```python
from build123d import *

# Parameters (mm, degrees)
F0_W     = 23.5877633095
F0_H     = 70.452131331
F0_R     = 11.8720680475
F1_DEPTH = 6


# Not quite as in the source:
# - a feature names something its author has since deleted; it is built from what else it names


with BuildPart() as f1:
    # F0 (on Front) → F1 (new body)
    with BuildSketch(Plane.XZ):
        with BuildLine():
            add(Edge.make_bspline(
                [(611.5972634537, -153.9022508941), (611.6433594367, -147.41064865), (611.6495089066, -143.6068529658), (611.6564787513, -143.3067750725)],
                knots=[235.725136676, 235.725136676, 235.725136676, 235.725136676, 267.1722290958, 267.1722290958, 267.1722290958, 267.1722290958], degree=3))
            Line((611.6564787513, -143.3067750725), (582.1564787513, -143.3067750725))
            Line((582.1564787513, -143.3067750725), (582.1564787513, -148.3067750725))
            Line((582.1564787513, -148.3067750725), (552.6564787513, -148.3067750725))
            Line((552.6564787513, -148.3067750725), (552.6564787513, -389.3067750725))
            Line((552.6564787513, -389.3067750725), (562.6564787513, -389.3067750725))
            Line((562.6564787513, -389.3067750725), (562.6564787513, -409.3067750725))
            Line((562.6564787513, -409.3067750725), (586.6564787513, -409.3067750725))
            add(Edge.make_bspline(
                [(586.6564787513, -409.3067750725), (608.6616471129, -402.2484026518), (611.2517312901, -202.5628331126), (611.5972634537, -153.9022508941)],
                knots=[0, 0, 0, 0, 235.725136676, 235.725136676, 235.725136676, 235.725136676], degree=3))
        make_face()
        with Locations((574.0745894078, -343.064654055)):
            Rectangle(F0_W, F0_H, mode=Mode.SUBTRACT)
        with Locations((580.0634622574, -230.3008177464)):
            Circle(F0_R, mode=Mode.SUBTRACT)
        with BuildLine():
            add(Edge.make_bspline(
                [(586.6564787513, 122.6932249275), (608.6616471129, 115.6348525069), (611.2517312901, -84.0507170322), (611.5972634537, -132.7112992508)],
                knots=[0, 0, 0, 0, 235.725136676, 235.725136676, 235.725136676, 235.725136676], degree=3))
            Line((586.6564787513, 122.6932249275), (562.6564787513, 122.6932249275))
            Line((562.6564787513, 122.6932249275), (562.6564787513, 102.6932249275))
            Line((562.6564787513, 102.6932249275), (552.6564787513, 102.6932249275))
            Line((552.6564787513, 102.6932249275), (552.6564787513, -138.3067750725))
            Line((552.6564787513, -138.3067750725), (582.1564787513, -138.3067750725))
            Line((582.1564787513, -138.3067750725), (582.1564787513, -143.3067750725))
            Line((582.1564787513, -143.3067750725), (611.6564787513, -143.3067750725))
            add(Edge.make_bspline(
                [(611.5972634537, -132.7112992508), (611.6433594367, -139.2029014949), (611.6495089066, -143.0066971792), (611.6564787513, -143.3067750725)],
                knots=[235.725136676, 235.725136676, 235.725136676, 235.725136676, 267.1722290958, 267.1722290958, 267.1722290958, 267.1722290958], degree=3))
        make_face()
        with Locations((580.0634622574, -56.3127323985)):
            Circle(F0_R, mode=Mode.SUBTRACT)
        with Locations((574.0745894078, 56.4511039101)):
            Rectangle(F0_W, F0_H, mode=Mode.SUBTRACT)
    extrude(amount=F1_DEPTH)


solid = f1.part
```
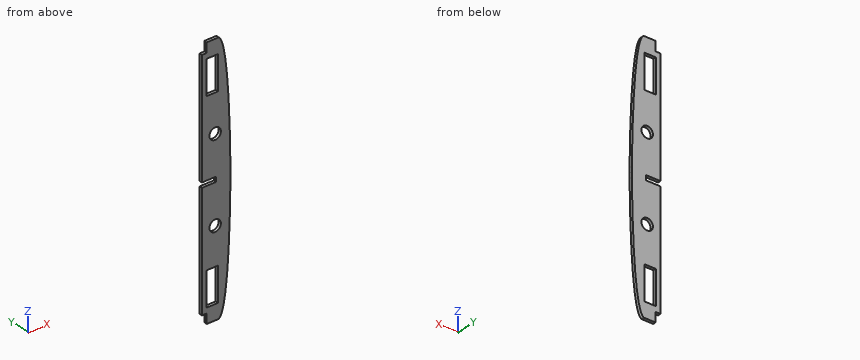
CAD build for the part. Positions are in the model's coordinates, mm. Coordinates: 2 decimals unless noted, no trailing zeros. Write each loop counter-clockwise with the first axis right and the second up, starting at its lowest first coordinate (ties: lowest second). Pieces come first, ordered by that corner, then holes. Notation, with made-up numbers: (-10, 17.5) -> (6, 17.5) arc R21 ccw to (6, 44.5) -> close; hole circle Ø11 at (27, -28.5). An arc over 180 degrees is marked (long way). Use CSV: the item, a comma, the result in double quotes. Start each with the question number.
Item 1: Drop flat-ended pins along their axis: P1, Ø1, axis at y = -3.5, z = -85, coming from the +X side; P2, Ø1, axis at x = 559.5, y = -5, coming from the -Z side; P3, Ø3, axis at y = -3.5, z = 110.5, coming from the -X side; P4, Ø19, axis at x = 580.06, z = -56.31, coming from the -Y side. Give the stop position or say it passes through.
Item 2: Band-saw the part on A-A, the plane x = 574. Write the cut outline in (y, z).
Item 3: Wall check: probe 1 along Z at (x, y) = (563.5, -0.5); probe 2 along Z at (x, y) = (561, -5); probe 3 along Z at (x, y) = (589, -3.5). Give the ranges that are in metal, low to high.
Item 4: Band-saw the part on B-B, the plane y = -5. Give the number of separate pieces and of enclosed holes in the cut face, plus the area to 3 significant figures.
Response values:
1,P1,"stops at x = 610.93"
1,P2,"stops at z = -389.31"
1,P3,"stops at x = 562.66"
1,P4,"passes through"
2,outline,"(-6, -409.31) -> (0, -409.31) -> (0, -378.29) -> (-6, -378.29) -> close; (-6, -307.84) -> (0, -307.84) -> (0, -240.51) -> (-6, -240.51) -> close; (-6, -220.09) -> (0, -220.09) -> (0, -148.31) -> (-6, -148.31) -> close; (-6, -138.31) -> (0, -138.31) -> (0, -66.52) -> (-6, -66.52) -> close; (-6, -46.11) -> (0, -46.11) -> (0, 21.23) -> (-6, 21.23) -> close; (-6, 91.68) -> (0, 91.68) -> (0, 122.69) -> (-6, 122.69) -> close"
3,probe 1,"z = -409.31 to -378.29, -307.84 to -148.31, -138.31 to 21.23, 91.68 to 122.69"
3,probe 2,"z = -389.31 to -148.31, -138.31 to 102.69"
3,probe 3,"z = -407.77 to -238.12, -222.49 to -64.13, -48.5 to 121.16"
4,separate pieces,"1"
4,enclosed holes,"4"
4,area,"23,700 mm2"
